Verification items for the finished model (mm, model axes). A direction names the side the tool comes from. Give positions to 0.01 mm unless a question says otherwise; leave off trailing zeros. Write each loop counter-clockwise with the first axis right and the second up, starting at its lowest first coordinate (ties: lowest second). Pieces come first, ordered by that corner, then holes. Notation, with made-up numbers: M 72.5,88.25 L 79.5,88.25 A33 ccw 79.5,116.25 Z; hole C 73,-25.75 d2. An arc over 180 degrees is marked long. Write item = value, one per line.
from build123d import *

# Parameters (mm, degrees)
ESBO_O1_W                = 6
ESBO_O1_H                = 12.4
ESBO_O1_W_2              = 10.4
ESBO_O1_R                = 1
ESBO_O1_R_2              = 2.5
RESSALTO_EXTRUS_O1_DEPTH = 18
CORTE_EXTRUS_O5_START    = 18
ESBO_O1_3_W              = 6
ESBO_O1_3_H              = 12.4
ESBO_O1_3_W_2            = 10.4
ESBO_O1_3_R              = 1
ESBO_O1_3_R_2            = 2.5
CORTE_EXTRUS_O5_DEPTH    = 34
ESBO_O3_R                = 1.05
ESBO_O3_W                = 1
ESBO_O3_H                = 5
CORTE_EXTRUS_O3_DEPTH    = 10
CORTE_EXTRUS_O4_DEPTH    = 2
ESBO_O5_R                = 1.65
CORTE_EXTRUS_O6_DEPTH    = 2.5
ESBO_O5_2_R              = 1.65
CORTE_EXTRUS_O7_DEPTH    = 5
FILETE1_R                = 3


with BuildPart() as part:
    # Esboço1 → Ressalto-extrusão1 (new body, symmetric)
    with BuildSketch(Plane.XY):
        Polygon((-1.4, -16.6), (-10.1, -9.4), (-10.1, 9.4), (10.1, 9.4), (10.1, -9.6), (2.1, -9.6), (2.1, -9.4), (0.1, -9.4), (0.1, -12.6), (10.1, -12.6), (10.1, -16.6), align=None)
        with Locations((-5.6, 0.4)):
            Rectangle(ESBO_O1_W, ESBO_O1_H, mode=Mode.SUBTRACT)
        with Locations((3.6, 0.4)):
            Rectangle(ESBO_O1_W_2, ESBO_O1_H, mode=Mode.SUBTRACT)
        with Locations((-5.6, 0.4)):
            Rectangle(ESBO_O1_W, ESBO_O1_H)
        with Locations((3.6, 0.4)):
            Rectangle(ESBO_O1_W_2, ESBO_O1_H)
        with Locations((3.6, 4.9)):
            Circle(ESBO_O1_R, mode=Mode.SUBTRACT)
        with Locations((3.6, -4.1)):
            Circle(ESBO_O1_R, mode=Mode.SUBTRACT)
        with Locations((3.6, 0.4)):
            Circle(ESBO_O1_R_2, mode=Mode.SUBTRACT)
    extrude(amount=RESSALTO_EXTRUS_O1_DEPTH, both=True)

    # Esboço1<3> → Corte-extrusão5 (cut)
    with BuildSketch(Plane.XY.offset(CORTE_EXTRUS_O5_START)):
        with Locations((-5.6, 0.4)):
            Rectangle(ESBO_O1_3_W, ESBO_O1_3_H)
        with Locations((3.6, 0.4)):
            Rectangle(ESBO_O1_3_W_2, ESBO_O1_3_H)
        with Locations((3.6, 4.9)):
            Circle(ESBO_O1_3_R, mode=Mode.SUBTRACT)
        with Locations((3.6, -4.1)):
            Circle(ESBO_O1_3_R, mode=Mode.SUBTRACT)
        with Locations((3.6, 0.4)):
            Circle(ESBO_O1_3_R_2, mode=Mode.SUBTRACT)
    extrude(amount=-CORTE_EXTRUS_O5_DEPTH, mode=Mode.SUBTRACT)

    # Esboço3 → Corte-extrusão3 (cut)
    with BuildSketch(Plane.XY.offset(18)):
        with Locations((-2.1, 7.65)):
            Circle(ESBO_O3_R)
        with Locations((-2.1, -7.3)):
            Circle(ESBO_O3_R)
        with Locations((-2.1, 0)):
            Rectangle(ESBO_O3_W, ESBO_O3_H)
    extrude(amount=-CORTE_EXTRUS_O3_DEPTH, mode=Mode.SUBTRACT)

    # Esboço4 → Corte-extrusão4 (cut)
    with BuildSketch(Plane.XY.offset(18)):
        with BuildLine():
            Line((-10.1, 9.4), (-10.1, -7.3))
            Line((-10.1, -7.3), (-4.1, -7.3))
            ThreePointArc((-4.1, -7.3), (-2.1, -9.3), (-0.1, -7.3))
            Line((-0.1, -7.3), (10.1, -7.3))
            Line((10.1, -7.3), (10.1, 9.4))
            Line((10.1, 9.4), (-10.1, 9.4))
        make_face()
    extrude(amount=-CORTE_EXTRUS_O4_DEPTH, mode=Mode.SUBTRACT)

    # Esboço5 → Corte-extrusão6 (cut)
    with BuildSketch(Plane(origin=(0, -12.6, 0), x_dir=(1, 0, 0), z_dir=(0, 1, 0))):
        Polygon((5.1, 6.535898385), (8.1, 8.267949192), (8.1, 11.732050808), (5.1, 13.464101615), (2.1, 11.732050808), (2.1, 8.267949192), align=None)
        with Locations((5.1, 10)):
            Circle(ESBO_O5_R, mode=Mode.SUBTRACT)
        Polygon((5.1, -13.464101615), (8.1, -11.732050808), (8.1, -8.267949192), (5.1, -6.535898385), (2.1, -8.267949192), (2.1, -11.732050808), align=None)
        with Locations((5.1, -10)):
            Circle(ESBO_O5_R, mode=Mode.SUBTRACT)
    extrude(amount=-CORTE_EXTRUS_O6_DEPTH, mode=Mode.SUBTRACT)

    # Esboço5<2> → Corte-extrusão7 (cut, through all)
    with BuildSketch(Plane(origin=(0, -12.6, 0), x_dir=(1, 0, 0), z_dir=(0, 1, 0))):
        with Locations((5.1, -10)):
            Circle(ESBO_O5_2_R)
        with Locations((5.1, 10)):
            Circle(ESBO_O5_2_R)
    extrude(amount=-CORTE_EXTRUS_O7_DEPTH, mode=Mode.SUBTRACT)

    # Filete1
    filete1_edges = [part.edges().sort_by_distance(p)[0] for p in [
        (-10.1, -9.4, 0),
        (-1.4, -16.6, 0),
    ]]
    fillet(filete1_edges, radius=FILETE1_R)


solid = part.part
1) Cross-section at A-A on y = 4.9. Record the boundary of the cut face in (x, z).
From the geometry:
outline = M -10.1,-18 L 2.6,-18 L 2.6,-16 L -1.6,-16 L -1.6,16 L -2.6,16 L -2.6,-16 L -8.6,-16 L -8.6,16 L -10.1,16 Z; M 4.6,-18 L 10.1,-18 L 10.1,16 L 8.8,16 L 8.8,-16 L 4.6,-16 Z
2) Cross-section at B-B on z = -15.5. Record the boundary of the cut face in (x, y).
From the geometry:
outline = M -10.1,-7.99 A3 ccw -9.01,-10.3 L -2.23,-15.91 A3 ccw -0.32,-16.6 L 10.1,-16.6 L 10.1,-12.6 L 0.1,-12.6 L 0.1,-9.4 L 2.1,-9.4 L 2.1,-9.6 L 10.1,-9.6 L 10.1,9.4 L -10.1,9.4 Z; hole M -8.6,-5.8 L -2.6,-5.8 L -2.6,6.6 L -8.6,6.6 Z; hole M -1.6,-5.8 L 8.8,-5.8 L 8.8,6.6 L -1.6,6.6 Z
3) Cross-section at D-D on x = -5.75. Record the boundary of the cut face in (y, z), plus the area to 3 significant figures.
From the geometry:
outline = M -13,-18 L 9.4,-18 L 9.4,16 L 6.6,16 L 6.6,-16 L -5.8,-16 L -5.8,16 L -7.3,16 L -7.3,18 L -13,18 Z
area = 376 mm^2
4) Depth check by flat-ended pin: P1, Ø3, axis at x = -5.5, z = -7.5, coming from the -Y side; P2, Ø5.5, axis at x = 3, y = -2, coming from the +Z side; P3, Ø3, axis at y = -12, z = -10.5, coming from the -X side. Enter the tip coordinate at first touch or a pass-through.
From the geometry:
P1 = -14.45
P2 = -16
P3 = -8.77
5) Draft check along X on faces 1 (the cylindrical face through (-9.8, -9.3, -0.3)), 2 (the flat face through (3.6, -13.8, -7.4)), 3 (the flat face through (0, -3, -18)), 4 (the flat face through (8.1, -14, -10)). Enter one of: +X half, -X half, draft (parallel to the pull), parting line (faces both ways), or undercut.
From the geometry:
face_1 = -X half
face_2 = undercut
face_3 = draft
face_4 = undercut
6) Cross-section at C-C on z = 10. Count the separate pieces of the cut face and the enclosed holes in it, plus the area to 3 significant figures.
From the geometry:
separate_pieces = 2
enclosed_holes = 3
area = 228 mm^2
7) Tool access check on faces 5 (the flat face through (-2, 0, 8)), 6 (the flat face through (0, -13, 18)), 7 (the flat face through (2.1, -14, 10)), 8 (the cylindrical face through (4.7, -15.8, -8.4)). Record the directions out of +Z, -Z, +X, -X, +Y, -Y that give a thin tool (end or side, any length) a straight path to the whole face; none if there is none.
From the geometry:
face_5 = +Z
face_6 = +Z, +X, -X, +Y, -Y
face_7 = none
face_8 = -Y
8) Material ranges on probe 1 along Y at (x, z) = (8, -8.5); probe 2 along Y at (x, z) = (3.75, -1); probe 3 along X at (y, z) = (3.75, 3), recorded low to high. Write a range as from..to.
From the geometry:
probe_1 = -16.6..-15.1, -9.6..-5.8, 6.6..9.4
probe_2 = -16.6..-12.6, -9.6..-5.8, 6.6..9.4
probe_3 = -10.1..-8.6, -2.6..-1.6, 8.8..10.1
